from build123d import *

# Parameters (mm, degrees)
F0_R     = 11
F0_R_2   = 4.5
F1_DEPTH = 7.8
F2_SIZE  = 0.2
F3_SIZE  = 2.75


with BuildPart() as f1:
    # F0 (on Top) → F1 (new body)
    with BuildSketch(Plane.XY):
        Circle(F0_R)
        Circle(F0_R_2, mode=Mode.SUBTRACT)
    extrude(amount=F1_DEPTH)

    # F2
    f2_edges = [f1.edges().sort_by_distance(p)[0] for p in [
        (-11, 0, 7.8),
        (-11, 0, 0),
        (-4.5, 0, 0),
    ]]
    chamfer(f2_edges, length=F2_SIZE)

    # F3
    f3_edges = [f1.edges().sort_by_distance(p)[0] for p in [
        (-4.5, 0, 7.8),
    ]]
    chamfer(f3_edges, length=F3_SIZE)


solid = f1.part
Geometry: final body of the model. Coordinates: model frame, mm. Round coordinates to 2 decimals unless told otherwise and drop trailing zeros. Loops run counter-clockwise (first coordinate to the right, second up) from the corner with the lowest first, then second, coordinate; pieces in that order, holes last. Notation, with made-up numbers: (51, 8) - (98, 8) arc R15 cw to (98, 23) - close; hole circle Ø6 at (-14.75, 35.25). An arc over 180 degrees is marked (long way). Write each question's results on one line, items separated by ' | '. Start each with the question number.
1) Mould query, pull axis Y, two halves, no side actions, for faces 1 (the face through (-0.59, 4.46, 2.59)), 2 (the face through (5, -2, 0)), 3 (the face through (-2.38, -10.74, 3.85)). Classes: released by +Y, released by -Y, zero draft, split by the parting line, or undercut.
2) First-contact query: P1, Ø2, axis at x = -6.5, z = 5, coming from the -Y side; P2, Ø2, axis at y = 3.5, z = 4, coming from the +X side; P3, Ø4, axis at x = 8.5, y = -8, coming from the +Z side; P4, Ø7, axis at x = 0, y = 0, coming from the +Z side. Flat tips, straight axial feed; report the tip coordinate or a pass-through.
3) Line query: probe 1 along Y at (x, z) = (0, 2.3); probe 2 along X at (y, z) = (-0.5, 2); probe 3 along Y at (x, z) = (-4, 2). Output: solid intervals per line, ascending. Write a range as [from, to].
4) Cut plane C-C on z = 2.5. Return loops of the section in (x, y), then the cut area to 3 significant figures.
5) Cut plane A-A on y = 0. Return loops of the section in (x, z), then the cut area to 3 significant figures.
Verdict:
1) face 1: undercut | face 2: zero draft | face 3: split by the parting line
2) P1: stops at y = -9.53 | P2: stops at x = 10.71 | P3: stops at z = 7.8 | P4: passes through
3) probe 1: y = [-11, -4.5], [4.5, 11] | probe 2: x = [-10.99, -4.47], [4.47, 10.99] | probe 3: y = [-10.25, -2.06], [2.06, 10.25]
4) outline: circle Ø22 at (0, 0); hole circle Ø9 at (0, 0) | area: 317 mm2
5) outline: (-11, 0.2) - (-10.8, 0) - (-4.7, 0) - (-4.5, 0.2) - (-4.5, 5.05) - (-7.25, 7.8) - (-10.8, 7.8) - (-11, 7.6) - close; (4.5, 0.2) - (4.7, 0) - (10.8, 0) - (11, 0.2) - (11, 7.6) - (10.8, 7.8) - (7.25, 7.8) - (4.5, 5.05) - close | area: 93.7 mm2
